Study the drawing (mm; zero at the part's minimum x, y, z) and answer. A direction names the side the tool comes from. Coordinates: 2 decimals unless noted, no trailing zeros. Loops run counter-clockwise (first coordinate to the right, second up) from the corner with the lowest first, then second, coordinate; pieces in that order, holes last. Notation, with made-up numbers: (26.5, 32.5) -> (59.5, 32.5) arc R11 cw to (59.5, 46.5) -> close; hole circle Ø10 at (27, 86.25). An arc over 180 degrees is marked (long way). Answer in a Markdown table with one row per item.
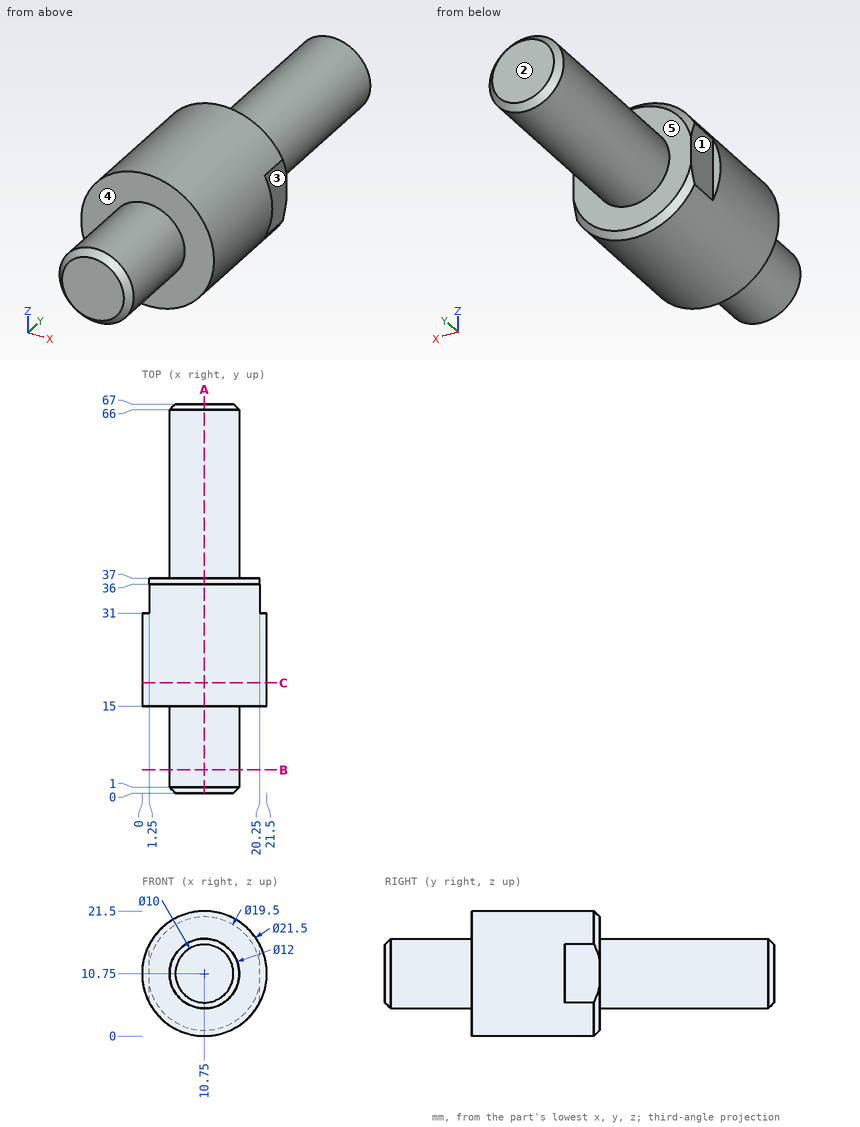
1. A cutting plane is placed at A-A on x = 10.75. Give the vertices of the cut face in (y, z).
A:
| item | result |
|---|---|
| outline | (0, 5.75) -> (1, 4.75) -> (15, 4.75) -> (15, 0) -> (36, 0) -> (37, 1) -> (37, 4.75) -> (66, 4.75) -> (67, 5.75) -> (67, 15.75) -> (66, 16.75) -> (37, 16.75) -> (37, 20.5) -> (36, 21.5) -> (15, 21.5) -> (15, 16.75) -> (1, 16.75) -> (0, 15.75) -> close |
2. A tool of negligible diameter and unlimited length cuts with its end or side. For the marked faces 1, 2, 3, 4 and 5, from which of +Z, -Z, +X, -X, +Y, -Y can it reach the whole face along a straight path? Write none if from no direction.
A:
| item | result |
|---|---|
| face 1 | +Z, -Z, -X, +Y |
| face 2 | +Z, -Z, +X, -X, +Y |
| face 3 | +Z, -Z, +X, +Y |
| face 4 | -Y |
| face 5 | +Y |
3. Given pin 1 Ø5 at (x, y) = (8, 16) entering from -Z; pin 2 Ø3 at (y, z) = (43.5, 4) entering from -X; pin 3 Ø3 at (y, z) = (33, 12) entering from -X; pin 4 Ø12 at (y, z) = (33, 16) entering from +X, each flat-ended and moving along its own axis, determine where each tip first touches the part or whether it passes through.
A:
| item | result |
|---|---|
| pin 1 | stops at z = 0 |
| pin 2 | stops at x = 7.85 |
| pin 3 | stops at x = 1.25 |
| pin 4 | stops at x = 21.5 |
4. Find the intervals of material crossed by probe 1 along Y at (x, z) = (18, 5.5); probe 2 along X at (y, z) = (5, 11); probe 3 along X at (y, z) = (24.5, 4.5), in increasing order.
A:
| item | result |
|---|---|
| probe 1 | y = 15 to 37 |
| probe 2 | x = 4.76 to 16.74 |
| probe 3 | x = 2 to 19.5 |
5. A cutting plane is placed at C-C on y = 19. Give the vertices of the cut face in (x, z).
A:
| item | result |
|---|---|
| outline | circle Ø21.5 at (10.75, 10.75) |
6. A cutting plane is placed at B-B on y = 4. Give the vertices of the cut face in (x, z).
A:
| item | result |
|---|---|
| outline | circle Ø12 at (10.75, 10.75) |
